Input: dimensioned drawing with shaded views. Units: mm. Origin: part minimum x, y, z. Round coordinates to 2 decimals unless told otherwise and drop trailing zeros. Loops run counter-clockwise (first coordinate to the right, second up) from the corner with the lowest first, then second, coordinate; pieces in that order, holes last. Notation, with made-up numbers: M 43.5,21 L 73.5,21 A27 cw 73.5,53 Z; hole C 38,57.5 d11. An arc over 180 degrees is marked long. Use one line per item in the form item = value. Start each with the question number.
Q1. Section query B-B, the plane y = 2.5. State how many separate pieces and enclosed holes the cut face has, and give its area (3 significant figures).
Q2. Ray query, line 1 along X through (y, z) = (1.65, 43.75); line 2 along X through (y, z) = (0.85, 67.25); line 3 along X through (y, z) = (0.7, 3). Return the intervals inside material, ascending.
Q3. Section query D-D, the plane x = 57. Output: boundary loops of the cut face in (y, z).
Q4. First-contact query: P1, Ø3.5, axis at x = 84, z = 23, coming from the -Y side. Flat tip, straight axial feed; report the tip coordinate or a pass-through.
Q5. Section query A-A, the plane x = 6. Output: boundary loops of the cut face in (y, z).
Q6. Section query C-C, the plane z = 3. Output: boundary loops of the cut face in (x, y), and give its area (3 significant figures).
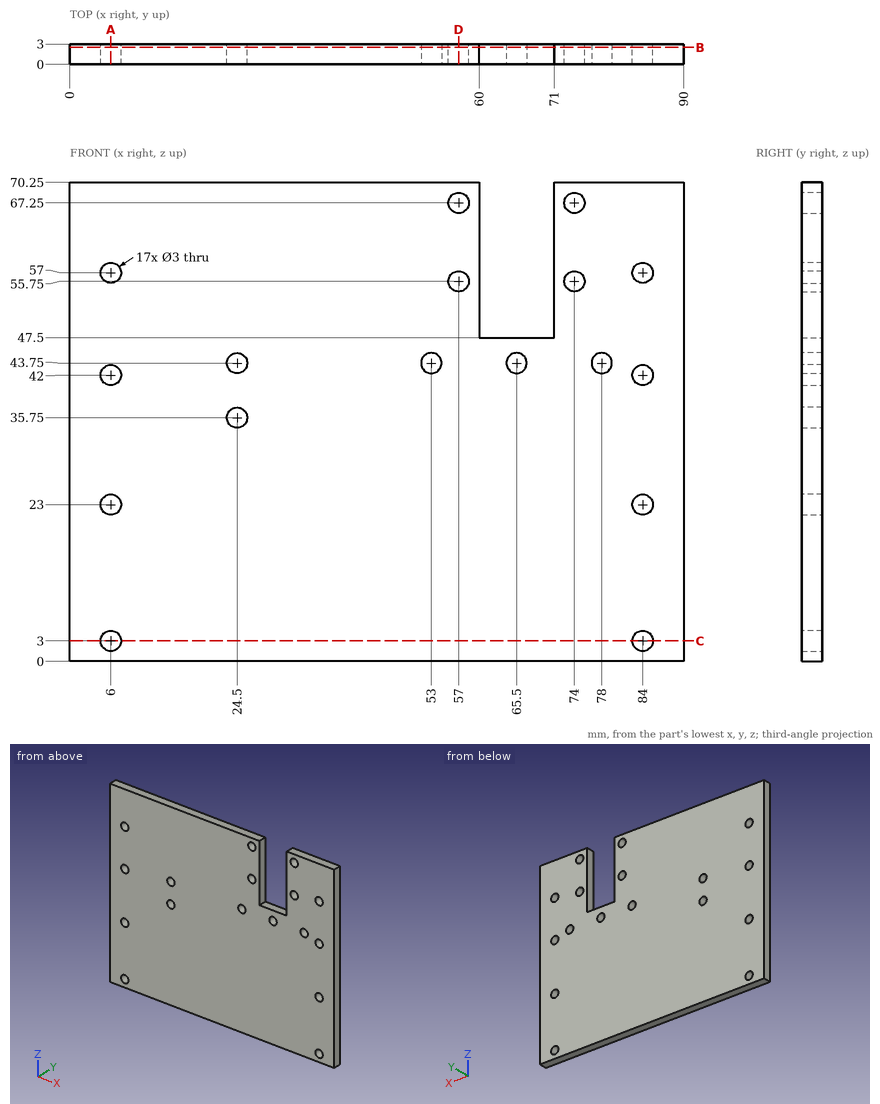
Results found:
q1.separate_pieces = 1
q1.enclosed_holes = 17
q1.area = 5,950 mm²
q2.line_1 = 0 to 23, 26 to 51.5, 54.5 to 64, 67 to 76.5, 79.5 to 90
q2.line_2 = 0 to 55.5, 58.5 to 60, 71 to 72.5, 75.5 to 90
q2.line_3 = 0 to 4.5, 7.5 to 82.5, 85.5 to 90
q3.outline = M 0,0 L 3,0 L 3,54.25 L 0,54.25 Z; M 0,57.25 L 3,57.25 L 3,65.75 L 0,65.75 Z; M 0,68.75 L 3,68.75 L 3,70.25 L 0,70.25 Z
q4.P1 = 0
q5.outline = M 0,0 L 3,0 L 3,1.5 L 0,1.5 Z; M 0,4.5 L 3,4.5 L 3,21.5 L 0,21.5 Z; M 0,24.5 L 3,24.5 L 3,40.5 L 0,40.5 Z; M 0,43.5 L 3,43.5 L 3,55.5 L 0,55.5 Z; M 0,58.5 L 3,58.5 L 3,70.25 L 0,70.25 Z
q6.outline = M 0,0 L 4.5,0 L 4.5,3 L 0,3 Z; M 7.5,0 L 82.5,0 L 82.5,3 L 7.5,3 Z; M 85.5,0 L 90,0 L 90,3 L 85.5,3 Z
q6.area = 252 mm²
